For this review, take the finished solid that the model builds, in its own axes (mm). A direction names the side the tool comes from. Round coordinates to 2 decimals unless told otherwise and drop trailing zeros. Write each loop counter-clockwise with the first axis right and the second up, starting at its lowest first coordinate (ties: lowest second). Pieces come first, ordered by that corner, then holes. Notation, with made-up numbers: (-33, 43.5) -> (-28, 43.5) arc R30 ccw to (-28, 79.5) -> close; hole circle Ø3 at (29.25, 82). An arc over 180 degrees is marked (long way). Answer as CSV lines item,"result". Start each with the question number.
Item 1: Take a section at A-A on y = 0. Give the boundary of the cut face in (x, z).
Item 2: Take a section at D-D on y = -56. Give the boundary of the cut face in (x, z).
Item 3: Machinability: for faces 5 (the flat face through (-12.7, -50, 3)), 6 (the flat face through (19, -24.892, 3)), 7 (the flat face through (15, -19, 5.08)), which of the approach directions +Z, -Z, +X, -X, +Y, -Y give a long, thin tool a straight path to every point of the face, cutting with its end or side? Answer none if there is none.
Item 4: Wall thickness on probe 1 along X at (y, z) = (-6.5, 4); probe 2 along Y at (x, z) = (-8, 2.65); probe 3 along X at (y, z) = (-15, 2.3): over which ranges is each line inside the solid? List them lowest first. Write a range as from..to.
Item 5: Mouldability with a two-part tool opening along X and no side actions: class faces 1 (the cylindrical face through (27.46, -7.34, 2.58)), 2 (the cylindrical face through (1.17, 35.54, 2.5)), 3 (the flat face through (12.7, -50, 3)), 4 (the cylindrical face through (-6.534, 27.863, 2.576)) as +X half, -X half, draft (parallel to the pull), parting line (faces both ways), or undercut.
Item 6: Take a section at C-C on z = 1.6. Give the boundary of the cut face in (x, y), then the cut area to 3 significant figures.
Item 7: For pin 1 Ø3.5 at (x, y) = (-24.26, -20.63) entering from +Z; pin 2 Ø1.5 at (x, z) = (-17.5, 1.5) entering from -Y, all flat-tipped, find the tip position at first contact; note any pin that passes through.
Item 8: Take a section at B-B on x = 0. Give the boundary of the cut face in (y, z), then the cut area to 3 significant figures.
```python
from build123d import *

# Parameters (mm, degrees)
SKETCH1_R           = 35.56
BOSS_EXTRUDE1_DEPTH = 5.08
CUT_EXTRUDE1_DEPTH  = 51.545361805
SKETCH7_R           = 2.032
CUT_EXTRUDE2_DEPTH  = 51.545361805
SKETCH8_R           = 21.336
CUT_EXTRUDE3_DEPTH  = 51.545361805
SKETCH9_W           = 25.4
SKETCH9_H           = 5.08
BOSS_EXTRUDE2_DEPTH = 50.8


with BuildPart() as part:
    # Sketch1 → Boss-Extrude1 (new body)
    with BuildSketch(Plane.XY):
        Circle(SKETCH1_R)
    extrude(amount=BOSS_EXTRUDE1_DEPTH)

    # Sketch2 → Cut-Extrude1 (cut, through all)
    with BuildSketch(Plane.XY.offset(5.08)):
        Polygon((0, -35.56), (-36.256055522, -35.56), (-36.256055522, -24.892), (33.75035888, -24.892), (33.75035888, -35.56), align=None)
    extrude(amount=-CUT_EXTRUDE1_DEPTH, mode=Mode.SUBTRACT)

    # Sketch7 → Cut-Extrude2 (cut, through all)
    with BuildSketch(Plane.XY.offset(5.08)):
        with Locations((-24.261099887, -20.626476503)):
            Circle(SKETCH7_R)
        with Locations((-7.471969114, 29.665523497)):
            Circle(SKETCH7_R)
        with Locations((25.522900113, -7.952823738)):
            Circle(SKETCH7_R)
    extrude(amount=-CUT_EXTRUDE2_DEPTH, mode=Mode.SUBTRACT)

    # Sketch8 → Cut-Extrude3 (cut, through all)
    with BuildSketch(Plane(origin=(0, 0, 0), x_dir=(-1, 0, 0), z_dir=(0, 0, -1))):
        Circle(SKETCH8_R)
    extrude(amount=-CUT_EXTRUDE3_DEPTH, mode=Mode.SUBTRACT)

    # Sketch9 → Boss-Extrude2 (add)
    with BuildSketch(Plane.XZ.offset(24.892)):
        with Locations((0, 2.54)):
            Rectangle(SKETCH9_W, SKETCH9_H)
    extrude(amount=BOSS_EXTRUDE2_DEPTH)


solid = part.part
```
Output values:
1,outline,"(-35.56, 0) -> (-21.34, 0) -> (-21.34, 5.08) -> (-35.56, 5.08) -> close; (21.34, 0) -> (35.56, 0) -> (35.56, 5.08) -> (21.34, 5.08) -> close"
2,outline,"(-12.7, 0) -> (12.7, 0) -> (12.7, 5.08) -> (-12.7, 5.08) -> close"
3,face 5,"+Z, -Z, -X, -Y"
3,face 6,"+Z, -Z, +X, -Y"
3,face 7,"+Z, +X, -X, +Y, -Y"
4,probe 1,"x = -34.96..-20.32, 20.32..24.1, 26.94..34.96"
4,probe 2,"y = -75.69..-19.78, 19.78..27.7, 31.63..34.65"
4,probe 3,"x = -32.24..-15.17, 15.17..32.24"
5,face 1,"undercut"
5,face 2,"parting line"
5,face 3,"+X half"
5,face 4,"undercut"
6,outline,"(-25.39, -24.89) -> (-12.7, -24.89) -> (-12.7, -75.69) -> (12.7, -75.69) -> (12.7, -24.89) -> (25.39, -24.89) arc R35.56 ccw (long way) to start; hole circle Ø4.06 at (-24.26, -20.63); hole circle Ø42.67 at (0, 0); hole circle Ø4.06 at (-7.47, 29.67); hole circle Ø4.06 at (25.52, -7.95)"
6,area,"3,420 mm^2"
7,pin 1,"passes through"
7,pin 2,"stops at y = -24.89"
8,outline,"(-75.69, 0) -> (-21.34, 0) -> (-21.34, 5.08) -> (-75.69, 5.08) -> close; (21.34, 0) -> (35.56, 0) -> (35.56, 5.08) -> (21.34, 5.08) -> close"
8,area,"348 mm^2"
